Check sheet for the modelled part. Datum: model origin and axes. Units: mm. A direction names the side the tool comes from. Round coordinates to 2 decimals unless told otherwise and drop trailing zeros. Write each loop counter-clockwise with the first axis right and the second up, starting at its lowest first coordinate (ties: lowest second). Pieces come first, ordered by that corner, then holes.
Item 1: Go/stop test with a flat-tipped pin: pin 1 Ø3.5 at (y, z) = (12, 1.5) entering from +X. Record where the tip stops, or that it passes through.
Item 2: Cross-section at A-A on z = 0. Enter the section's corners in (x, y), plus the area to 3 significant figures.
Item 3: Tool access check on faces 1 (the flat face through (81, 11, 0)), 2 (the flat face through (-2, 10, -43)). Record the directions out of +Z, -Z, +X, -X, +Y, -Y that give a thin tool (end or side, any length) a straight path to the whole face; none if there is none.
Item 4: Release check for a two-part mould opening along Y. For faces 3 (the flat face through (-2, -14, 1)), 4 (the flat face through (111, 4.7, 0.6)), 5 (the cylindrical face through (96.21, 5.143, 1.301)) record: +Y half, -Y half, draft (parallel to the pull), parting line (faces both ways), or undercut.
Item 5: Cross-section at B-B on y = 11. Enter the section's corners in (x, z), plus the area to 3 significant figures.
Item 6: Material ranges on line 1 (Y direction, x = 88, z = 0); line 2 (X direction, y = 7.5, z = 3.5); line 3 (Z direction, x = 99.5, y = 9.5), recorded low to high.
from build123d import *

# Parameters (mm, degrees)
SKETCH1_W           = 222
SKETCH1_H           = 86
BOSS_EXTRUDE1_DEPTH = 22
SKETCH2_R           = 6
CUT_EXTRUDE1_DEPTH  = 30
SKETCH3_W           = 222
SKETCH3_H           = 86
BOSS_EXTRUDE2_DEPTH = 14
SKETCH4_W           = 222
SKETCH4_H           = 86
BOSS_EXTRUDE3_DEPTH = 13


with BuildPart() as part:
    # Sketch1 → Boss-Extrude1 (new body)
    with BuildSketch(Plane(origin=(0, 0, 0), x_dir=(1, 0, 0), z_dir=(0, 1, 0))):
        Rectangle(SKETCH1_W, SKETCH1_H)
    extrude(amount=BOSS_EXTRUDE1_DEPTH)

    # Sketch2 → Cut-Extrude1 (cut)
    with BuildSketch(Plane(origin=(111, 0, 0), x_dir=(0, 0, -1), z_dir=(1, 0, 0))):
        with Locations((0, 11)):
            Circle(SKETCH2_R)
    extrude(amount=-CUT_EXTRUDE1_DEPTH, mode=Mode.SUBTRACT)

    # Sketch3 → Boss-Extrude2 (add)
    with BuildSketch(Plane.XZ):
        Rectangle(SKETCH3_W, SKETCH3_H)
    extrude(amount=BOSS_EXTRUDE2_DEPTH)

    # Sketch4 → Boss-Extrude3 (add)
    with BuildSketch(Plane(origin=(0, 22, 0), x_dir=(1, 0, 0), z_dir=(0, 1, 0))):
        Rectangle(SKETCH4_W, SKETCH4_H)
    extrude(amount=BOSS_EXTRUDE3_DEPTH)


solid = part.part
Response values:
1. pin 1: stops at x = 81
2. outline: (-111, -14) - (111, -14) - (111, 5) - (81, 5) - (81, 17) - (111, 17) - (111, 35) - (-111, 35) - close
2. area: 10,500 mm2
3. face 1: +X
3. face 2: -Z, +X, -X, +Y, -Y
4. face 3: -Y half
4. face 4: draft
4. face 5: undercut
5. outline: (-111, -43) - (111, -43) - (111, -6) - (81, -6) - (81, 6) - (111, 6) - (111, 43) - (-111, 43) - close
5. area: 18,700 mm2
6. line 1: y = -14 to 5, 17 to 35
6. line 2: x = -111 to 81
6. line 3: z = -43 to -5.81, 5.81 to 43
